For this review, use the dimensioned drawing (mm, ordinates from the lowest corner) and the shaded views. Give positions to 0.01 mm unless a question says otherwise; leave off trailing zeros. Order: outer loops, then holes, each group sorted by start corner. A loop starts at its lowest first (then second) coordinate and runs counter-clockwise, first axis right, second up. Notation, with made-up numbers: (85.5, -32) - (130.5, -32) arc R21 cw to (130.5, -2) - close; hole circle Ø9 at (2.5, -35.5). An arc over 180 degrees is marked (long way). Use a Markdown table: item, result. Add a question column.
1) We need section B-B on y = 5.5. Write out the cut boundary in (x, z), then the cut area to 3 significant figures.
2) Wall thickness on L1, parallel to Y at x = 70, z = 1.5; L2, parallel to Y at x = 42.5, z = 1.85; L3, parallel to X at y = 9, z = 2.1: over which ranges is each line inside the solid? List them lowest first.
3) Clearance check with flat-ended pins moving along their axes: P1, Ø5.5, axis at x = 42.5, y = 10, coming from the -Z side; P2, Ø12, axis at x = 48, y = 5, coming from the -Z side. State where each tip first meets the part, or that it passes through.
4) We need section C-C on z = 1.95. Write out the cut boundary in (x, y).
5) We need section A-A on x = 70. Write out the cut boundary in (y, z), then the cut area to 3 significant figures.
6) We need section D-D on y = 9. Write out the cut boundary in (x, z), then the cut area to 3 significant figures.
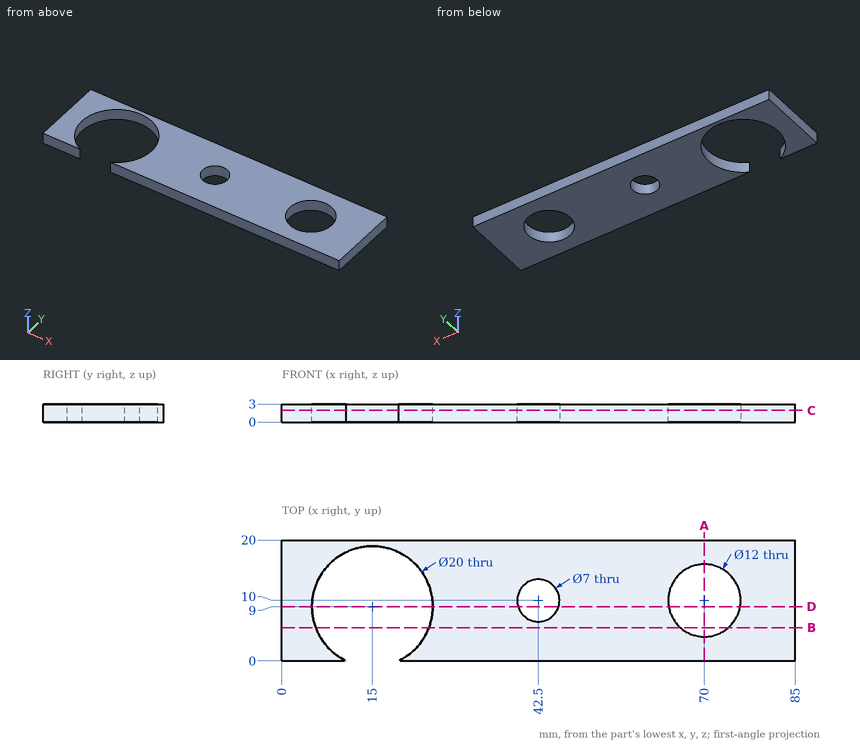
Checked values:
| question | item | result |
|---|---|---|
| 1 | outline | (0, 0) - (5.63, 0) - (5.63, 3) - (0, 3) - close; (24.37, 0) - (66.03, 0) - (66.03, 3) - (24.37, 3) - close; (73.97, 0) - (85, 0) - (85, 3) - (73.97, 3) - close |
| 1 | area | 175 mm² |
| 2 | L1 | 0 to 4, 16 to 20 |
| 2 | L2 | 0 to 6.5, 13.5 to 20 |
| 2 | L3 | 0 to 5, 25 to 39.15, 45.85 to 64.08, 75.92 to 85 |
| 3 | P1 | through |
| 3 | P2 | z = 0 |
| 4 | outline | (0, 0) - (10.64, 0) arc R10 cw (long way) to (19.36, 0) - (85, 0) - (85, 20) - (0, 20) - close; hole circle Ø7 at (42.5, 10); hole circle Ø12 at (70, 10) |
| 5 | outline | (0, 0) - (4, 0) - (4, 3) - (0, 3) - close; (16, 0) - (20, 0) - (20, 3) - (16, 3) - close |
| 5 | area | 24.0 mm² |
| 6 | outline | (0, 0) - (5, 0) - (5, 3) - (0, 3) - close; (25, 0) - (39.15, 0) - (39.15, 3) - (25, 3) - close; (45.85, 0) - (64.08, 0) - (64.08, 3) - (45.85, 3) - close; (75.92, 0) - (85, 0) - (85, 3) - (75.92, 3) - close |
| 6 | area | 139 mm² |
